Autodesk Inventor part; units mm, degrees
ref_plane "YZ Plane" through (0, 0, 0) normal (1, 0, 0) x (0, 1, 0)
ref_plane "XZ Plane" through (0, 0, 0) normal (0, 1, 0) x (-1, 0, 0)
ref_plane "XY Plane" through (0, 0, 0) normal (0, 0, 1) x (1, 0, 0)
sketch "Sketch1" plane through (0, 0, 0) normal (0, 1, 0) x (-1, 0, 0)
  line L0 (0, 0) -> (17, 0)
  circle A0 centre (0, 0) radius 17
  dimension "d0" = 17
extrude "Extrusion1" add sketch "Sketch1" along normal blind 2
sketch "Sketch2" plane through (0, 2, 0) normal (0, 1, 0) x (1, 0, 0)
  line L0 (0, 0) -> (-15, 0)
  circle A0 centre (0, 0) radius 15
  dimension "d3" = 15
extrude "Extrusion2" add sketch "Sketch2" along normal blind 4.8
sketch "Sketch3" plane through (0, 6.8, 0) normal (0, 1, 0) x (1, 0, 0)
  circle A0 centre (0, 0) radius 17
extrude "Extrusion3" add sketch "Sketch3" along normal blind 2
fillet "Fillet1" radius 2 2 edges at (-17, 8.8, 0) (17, 0, 0)
chamfer "Chamfer1" distance 1 angle 45 4 edges at (-17, 6.8005, 0) (-17, 6.8, 0) (17, 2, 0) (17, 1.9995, 0)
sketch "Sketch4" plane through (0, 8.8, 0) normal (0, 1, 0) x (1, 0, 0)
  circle A0 centre (0, 0) radius 13.75
  circle A1 centre (0, 0) radius 5
  dimension "d12" = 27.5
  dimension "d13" = 10
extrude "Extrusion4" cut sketch "Sketch4" against normal blind 1.5
fillet "Fillet2" radius 1.2 1 edges at (-13.75, 8.8, 0)
fillet "Fillet3" radius 1.5 1 edges at (-5, 8.8, 0)
sketch "Sketch5" plane through (0, 8.8, 0) normal (0, 1, 0) x (1, 0, 0)
  circle A0 centre (0, 0) radius 3.5
  circle A1 centre (0, 0) radius 3
  dimension "d18" = 6
extrude "Extrusion5" cut sketch "Sketch5" against normal blind 3.2 contours A1
sketch "Sketch6" plane through (0, 5.6, 0) normal (0, 1, 0) x (1, 0, 0)
  circle A0 centre (0, 0) radius 2
  dimension "d21" = 4
extrude "Extrusion6" cut sketch "Sketch6" against normal blind 5
sketch "Sketch7" plane through (0, 0.6, 0) normal (0, 1, 0) x (1, 0, 0)
  circle A0 centre (0, 0) radius 2
  line L0 (0, -2) -> (-2, 0)
  line L1 (-2, 0) -> (0, 2)
  line L2 (0, 2) -> (2, 0)
  line L3 (2, 0) -> (0, -2)
  line L4 (0, 2.2828) -> (-2.2828, 0)
  line L5 (-2.2828, 0) -> (0, -2.2828)
  line L6 (0, -2.2828) -> (2.2828, 0)
  line L7 (2.2828, 0) -> (0, 2.2828)
  point P0 (1.9764, 0.3065)
  point P1 (0.3065, 1.9764)
  point P2 (0.3065, -1.9764)
  point P3 (1.9764, -0.3065)
  point P4 (-0.3065, 1.9764)
  point P5 (-1.9764, 0.3065)
  point P6 (-1.9764, -0.3065)
  point P7 (-0.3065, -1.9764)
  dimension "d26" = 0.2
extrude "Extrusion7" cut sketch "Sketch7" against normal blind 5 contours L2 A0 L7 | L3 L0 L1 L2 | A0 L6 L3 | L1 A0 L4 | A0 L5 L0
properties part number "kolo_mensi"
Could you check a few things on this model? Use its own coordinates, in mm. A direction names the side the tool comes from. Coordinates: 2 decimals unless noted, no trailing zeros. Order: outer loops, then holes, each group sorted by start corner. A loop starts at its lowest first (then second) coordinate and runs counter-clockwise, first axis right, second up. Notation, with made-up numbers: M 6.25,65 L 54.25,65 A27 ccw 54.25,99 Z; hole C 21.25,24 d1. An arc over 180 degrees is marked long. Use a Markdown table: item, result. Add a question column.
Q1. If I drill on L1, parallel to Z at x = 0, y = 7.4; L2, parallel to X at y = 7.45, z = 0; L3, parallel to X at y = 3.5, z = 1.5, over which ranges is the centre line in solid material (lowest first)?
Q2. Which directions (+Z, -Z, +X, -X, +Y, -Y) give clear straight access to the entire face, cutting with the end or side of a thin tool? Please do faces 1 (the cylindrical face through (-14.985, 4.366, 0.66)), 2 (the flat face through (-1.13, 0.3, -1.15)), 3 (the flat face through (1, 5.6, 2)).
Q3. I want a section at A-A on y = 3.5. List the corners of the cut face in (x, z) for me, then the cut area to 3 significant figures.
Q4. I'm going to push flat-ended pins straight in: pin 1 (1.8 mm diameter, centred on x = 1, z = -1, fed in from +Y); pin 2 (4 mm diameter, centred on y = 3.5, z = -1, fed in from -X); pin 3 (3 mm diameter, centred on x = 0, z = 0, fed in from -Y); pin 4 (1 mm diameter, centred on y = 7, z = -6, fed in from -X). Where does each tip first touch, or does it pass through?
Q5. We'd pull the mould along Y, two halves only. Please class faces 4 (the flat face through (1.15, 0.3, -1.13)), 5 (the flat face through (-1.3, 0.6, 1.3)), 6 (the flat face through (-14, 2, 6)): pulls with the +Y half, pulls with the -Y half, needs draft (parallel to the pull), parting line crosses it, or undercut.
Checked values:
| question | item | result |
|---|---|---|
| 1 | L1 | -16.46 to -13.75, -5 to -3, 3 to 5, 13.75 to 16.46 |
| 1 | L2 | -16.5 to -13.75, -4.99 to -3, 3 to 4.99, 13.75 to 16.5 |
| 1 | L3 | -14.92 to -1.32, 1.32 to 14.92 |
| 2 | face 1 | none |
| 2 | face 2 | +Y, -Y |
| 2 | face 3 | +Y |
| 3 | outline | C 0,0 d30; hole C 0,0 d4 |
| 3 | area | 694 mm² |
| 4 | pin 1 | y = 5.6 |
| 4 | pin 2 | x = -16.36 |
| 4 | pin 3 | through |
| 4 | pin 4 | x = -15.46 |
| 5 | face 4 | needs draft |
| 5 | face 5 | pulls with the +Y half |
| 5 | face 6 | undercut |
